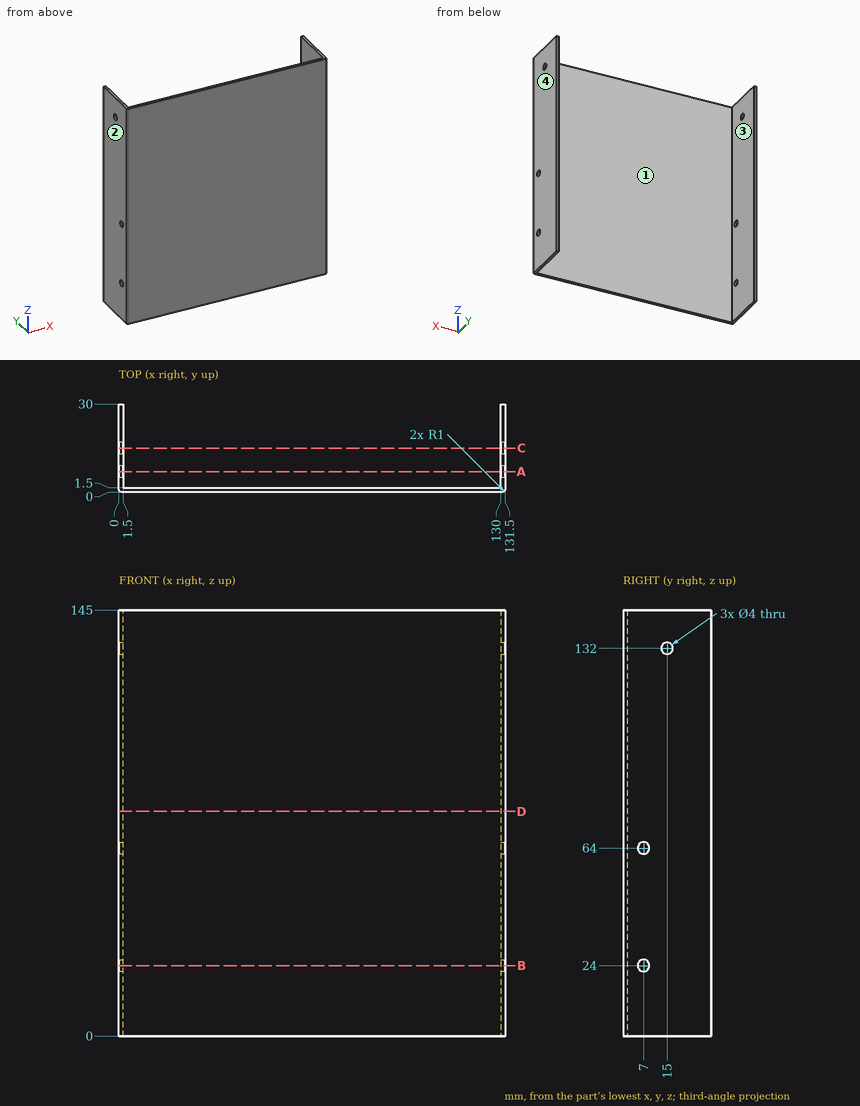
Geometry: see drawing. Coordinates: mm, zero at the bounding-box minimum. Coordinates: 2 decimals unless noted, no trailing zeros. Loops run counter-clockwise (first coordinate to the right, second up) from the corner with the lowest first, then second, coordinate; pieces in that order, holes last. Notation, with made-up numbers: M 63.5,3 L 117.5,3 A17 cw 117.5,18 Z; hole C 66,36 d10. An arc over 180 degrees is marked long. Answer in a Markdown table with one row per item.
1. Section A-A, the plane y = 7. Output: boundary loops of the cut face in (x, z).
Response:
| item | result |
|---|---|
| outline | M 0,0 L 1.5,0 L 1.5,22 L 0,22 Z; M 0,26 L 1.5,26 L 1.5,62 L 0,62 Z; M 0,66 L 1.5,66 L 1.5,145 L 0,145 Z; M 130,0 L 131.5,0 L 131.5,22 L 130,22 Z; M 130,26 L 131.5,26 L 131.5,62 L 130,62 Z; M 130,66 L 131.5,66 L 131.5,145 L 130,145 Z |
2. Section B-B, the plane z = 24. Output: boundary loops of the cut face in (x, y).
Response:
| item | result |
|---|---|
| outline | M 0,1 A1 ccw 1,0 L 130.5,0 A1 ccw 131.5,1 L 131.5,5 L 130,5 L 130,1.5 L 1.5,1.5 L 1.5,5 L 0,5 Z; M 0,9 L 1.5,9 L 1.5,30 L 0,30 Z; M 130,9 L 131.5,9 L 131.5,30 L 130,30 Z |
3. Draft query along X for the marked faces 1, 2, 3 and 4. Return one class per face: pulls with the +X half, pulls with the -X half, needs draft (parallel to the pull), parting line crosses it, or undercut.
Response:
| item | result |
|---|---|
| face 1 | undercut |
| face 2 | pulls with the -X half |
| face 3 | undercut |
| face 4 | pulls with the +X half |
4. Material intervals for line 1 (Z direction, x = 1.1, y = 7); line 2 (X direction, y = 21.5, z = 34.5); line 3 (Z direction, x = 0.3, y = 15), sorted ascending.
Response:
| item | result |
|---|---|
| line 1 | z = 0 to 22, 26 to 62, 66 to 145 |
| line 2 | x = 0 to 1.5, 130 to 131.5 |
| line 3 | z = 0 to 130, 134 to 145 |
5. Section C-C, the plane y = 15. Output: boundary loops of the cut face in (x, z), then the cut area to 3 significant figures.
Response:
| item | result |
|---|---|
| outline | M 0,0 L 1.5,0 L 1.5,130 L 0,130 Z; M 0,134 L 1.5,134 L 1.5,145 L 0,145 Z; M 130,0 L 131.5,0 L 131.5,130 L 130,130 Z; M 130,134 L 131.5,134 L 131.5,145 L 130,145 Z |
| area | 423 mm2 |
6. Section D-D, the plane z = 76.5. Output: boundary loops of the cut face in (x, y).
Response:
| item | result |
|---|---|
| outline | M 0,1 A1 ccw 1,0 L 130.5,0 A1 ccw 131.5,1 L 131.5,30 L 130,30 L 130,1.5 L 1.5,1.5 L 1.5,30 L 0,30 Z |
